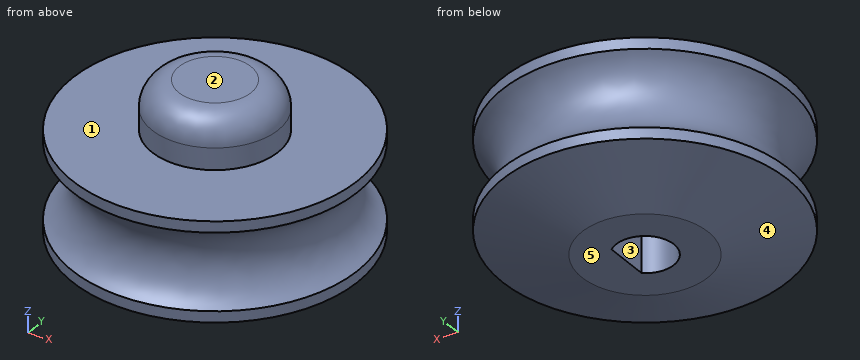
```python
from build123d import *

# Parameters (mm, degrees)
SKETCH_1_R          = 7.9
EXTRUDE_1_DEPTH     = 5.5
SKETCH_2_R          = 3.5
EXTRUDE_2_DEPTH     = 2.7
CUT_EXTRUDE_1_DEPTH = 9.3
FILLET_1_R          = 1.5


with BuildPart() as part:
    # 스케치1 → 보스-돌출1 (new body)
    with BuildSketch(Plane.XY):
        Circle(SKETCH_1_R)
    extrude(amount=EXTRUDE_1_DEPTH)

    # 스케치2 → 보스-돌출2 (add)
    with BuildSketch(Plane.XY.offset(5.5)):
        Circle(SKETCH_2_R)
    extrude(amount=EXTRUDE_2_DEPTH)

    # 스케치6 → 회전1 (revolve)
    with BuildSketch(Plane(origin=(0, 0, 0), x_dir=(0, 0, -1), z_dir=(1, 0, 0))):
        Polygon((0, -7.9), (1.303339378, -3.5), (1.303339378, 0), (0, 0), align=None)
    revolve(axis=Axis((0, 0, 0), (0, 0, -1)))

    # 스케치7 → 컷-돌출1 (cut)
    with BuildSketch(Plane(origin=(0, 0, -1.303339378), x_dir=(-1, 0, 0), z_dir=(0, 0, -1))):
        with BuildLine():
            ThreePointArc((1.6, 0), (0.681175455, 1.447756886), (-1.02, 1.232720568))
            Line((-1.02, 1.232720568), (-1.02, -1.232720568))
            ThreePointArc((-1.02, -1.232720568), (0.681175455, -1.447756886), (1.6, 0))
        make_face()
    extrude(amount=-CUT_EXTRUDE_1_DEPTH, mode=Mode.SUBTRACT)

    # 필렛1
    fillet_1_edges = [part.edges().sort_by_distance(p)[0] for p in [
        (-3.5, 0, 8.2),
    ]]
    fillet(fillet_1_edges, radius=FILLET_1_R)

    # 스케치8 → 컷-회전1 (revolve, cut)
    with BuildSketch(Plane(origin=(0, 0, 0), x_dir=(0, 0, -1), z_dir=(1, 0, 0))):
        with BuildLine():
            Line((-4.885, 7.9), (-0.615, 7.9))
            ThreePointArc((-0.615, 7.9), (-2.75, 6.700682513), (-4.885, 7.9))
        make_face()
    revolve(axis=Axis((0, 0, 0), (0, 0, 1)), mode=Mode.SUBTRACT)


solid = part.part
```
The listing builds one solid part. Answer for the finished solid, in the listing's coordinates (mm). Face numbers are marked on the shaded views. A direction names the side the tool comes from. Give positions to 0.01 mm unless a question says otherwise; leave off trailing zeros. Loops run counter-clockwise (first coordinate to the right, second up) from the corner with the lowest first, then second, coordinate; pieces in that order, holes last. Notation, with made-up numbers: (-8, 7.25) - (7, 7.25) arc R28 cw to (7, 30.25) - close; hole circle Ø10 at (26.5, 16.5). An arc over 180 degrees is marked (long way). Return JSON: item names as keys, results as strings. Group by question number.
1. Which of the six approach directions +Z, -Z, +X, -X, +Y, -Y give full straight-line access (tool end or side, diameter ignored) to the marked faces 1 and 2?
2. Straight lines are drawn through the part: line 1 (X direction, y = 0.5, z = 2); line 2 (X direction, y = -0.25, z = 1); line 3 (Z direction, x = 6.25, y = -3). For each, find the intervals that lie inside material, in ascending order. Write a range as [from, to].
3. Find section B-B (z = 1). Write down the section's boundary in (x, y).
4. Given pin 1 Ø4 at (x, y) = (2, 4.5) entering from +Z; pin 2 Ø1.3 at (x, y) = (0, -0.5) entering from -Z; pin 3 Ø1.5 at (y, z) = (-0.5, 1.5) entering from +X, each flat-ended and moving along its own axis, determine where each tip first touches the part or whether it passes through.
5. Determine the mould class of the marked faces 3, 4 and 5 for opening direction X: pulls with the +X half, pulls with the -X half, needs draft (parallel to the pull), parting line crosses it, or undercut.
6. Find section A-A (x = 0). Write down the section's boundary in (y, z) (3 decimals), then the cut area to 3 significant figures.
7. Find section C-C (z = 7). Write down the section's boundary in (x, y).
Verdict:
{
 "1": {"face 1": "+Z", "face 2": "+Z, +X, -X, +Y, -Y"},
 "2": {"line 1": "x = [-6.8, -1.52], [1.02, 6.8]", "line 2": "x = [-7.41, -1.58], [1.02, 7.41]", "line 3": "z = [-0.29, 1.7], [3.8, 5.5]"},
 "3": {"outline": "circle Ø14.83 at (0, 0); hole (1.02, -1.23) - (1.02, 1.23) arc R1.6 ccw (long way) to start"},
 "4": {"pin 1": "stops at z = 7.88", "pin 2": "stops at z = 8", "pin 3": "stops at x = 7.69"},
 "5": {"face 3": "undercut", "face 4": "parting line crosses it", "face 5": "needs draft"},
 "6": {"outline": "(-7.9, 0) - (-3.5, -1.303) - (-1.6, -1.303) - (-1.6, 7.997) - (1.6, 7.997) - (1.6, -1.303) - (3.5, -1.303) - (7.9, 0) - (7.9, 0.615) arc R2.5 cw to (7.9, 4.885) - (7.9, 5.5) - (3.5, 5.5) - (3.5, 6.7) arc R1.5 ccw to (2, 8.2) - (-2, 8.2) arc R1.5 ccw to (-3.5, 6.7) - (-3.5, 5.5) - (-7.9, 5.5) - (-7.9, 4.885) arc R2.5 cw to (-7.9, 0.615) - close", "area": "82.7 mm^2"},
 "7": {"outline": "circle Ø6.94 at (0, 0); hole (1.02, -1.23) - (1.02, 1.23) arc R1.6 ccw (long way) to start"}
}
